Can you work these out from the model? Positions are in its coordinate system, mm. A direction names the side the tool comes from. Coordinates: 2 decimals unless noted, no trailing zeros. Order: outer loops, then holes, each group sorted by start corner. A loop starts at its lowest first (then second) coordinate and runs counter-clockwise, first axis right, second up. Notation, with made-up numbers: M 70,-11 L 80,-11 A13 cw 80,9 Z; hole C 40.25,76 d10. An arc over 180 degrees is marked long. Answer as CSV lines item,"result". Start each with the question number.
1. On a 3-axis mill with a long thin cutter (end or side, diameter ignored), from which of +Z, -Z, +X, -X, +Y, -Y can I reach the whole of each face in a straight line? I mean faces 5 (the face through (-0.631, -1.479, 92.056)), 6 (the face through (-55, -3, 40)), 7 (the face through (-121.908, -1.479, 1.504)). Say none if no direction works.
2. If we section it at D-D (z = 98): List the corners of the cut face in (x, y) for me, plus the area to 3 significant figures.
3. If we section it at A-A (z = 38): List the corners of the cut face in (x, y) for me, plus the area to 3 significant figures.
4. If we section it at C-C (x = -72): List the corners of the cut face in (y, z) for me.
5. Will these pins go through, and if not, where does the flat tip stop? pin 1 (1.5 mm diameter, centred on y = -2, z = 54.5, fed in from +X); pin 2 (1.5 mm diameter, centred on y = -1.5, z = 49, fed in from -X); pin 3 (1.5 mm diameter, centred on y = -2, z = 15.5, fed in from -X).
6. If we mould it in two halves opening along X, with no side actions, what happens to faces 1 (the face through (12.443, -1.479, 67.745)), 2 (the face through (-55, 0, 40)), 3 (the face through (-154.63, -1.48, 7.35)), 4 (the face through (45.943, -1.479, 87.404))? For each: released by +X, released by -X, zero draft, split by the parting line, or undercut.
7. I need wall thicknesses on line 1 along X through (y, z) = (-2, 72); line 2 along X through (y, z) = (-1.35, 34); line 3 along X through (y, z) = (-1, 64.5). Which ranges of each line are inside material? Lowest first, please. Write a range as from..to.
```python
from build123d import *

# Parameters (mm, degrees)
F1_DEPTH = 3


with BuildPart() as f1:
    # F0 (on Front) → F1 (new body)
    with BuildSketch(Plane.XZ):
        with BuildLine():
            Line((-20, 0), (-5, 0))
            ThreePointArc((-5, 0), (-1.464466, 1.464466), (0, 5))
            Line((0, 5), (0, 60))
            Line((0, 60), (25.2391, 75.709675))
            ThreePointArc((25.2391, 75.709675), (39.261161, 56.50437), (57.673644, 71.552373))
            Line((57.673644, 71.552373), (57.576732, 71.481567))
            Line((57.576732, 71.481567), (33.979088, 103.779418))
            Line((33.979088, 103.779418), (29.703019, 111.034036))
            Line((29.703019, 111.034036), (25.755882, 103.779418))
            Line((25.755882, 103.779418), (20.821964, 111.527428))
            Line((20.821964, 111.527428), (18.203917, 103.779418))
            Line((18.203917, 103.779418), (-20, 80))
            Line((-20, 80), (-120, 80))
            Line((-120, 80), (-132.250323, 93.696277))
            ThreePointArc((-132.250323, 93.696277), (-139.249154, 95.394938), (-143.333333, 89.462944))
            Line((-143.333333, 89.462944), (-143.333333, 9.462944))
            Line((-143.333333, 9.462944), (-156.787529, 25.438112))
            ThreePointArc((-156.787529, 25.438112), (-158.470845, 26.310515), (-160.278011, 25.737113))
            Line((-160.278011, 25.737113), (-164.137305, 22.486838))
            ThreePointArc((-164.137305, 22.486838), (-165.009708, 20.803522), (-164.436306, 18.996356))
            Line((-164.436306, 18.996356), (-144.540306, -4.627645))
            ThreePointArc((-144.540306, -4.627645), (-137.506096, -6.502206), (-133.333333, -0.53713))
            Line((-133.333333, -0.53713), (-133.333333, 82.907007))
            Line((-133.333333, 82.907007), (-123.333333, 71.726667))
            Line((-123.333333, 71.726667), (-123.333333, 5))
            ThreePointArc((-123.333333, 5), (-121.868867, 1.464466), (-118.333333, 0))
            Line((-118.333333, 0), (-103.333333, 0))
            Line((-103.333333, 0), (-103.333333, 25))
            Line((-103.333333, 25), (-100.333333, 25))
            Line((-100.333333, 25), (-100.333333, 0))
            Line((-100.333333, 0), (-23, 0))
            Line((-23, 0), (-23, 25))
            Line((-23, 25), (-20, 25))
            Line((-20, 25), (-20, 0))
        make_face()
    extrude(amount=F1_DEPTH)


solid = f1.part
```
Solved:
1,face 5,"+Z, +Y, -Y"
1,face 6,"+Z, -Z, +X, -X, -Y"
1,face 7,"-Z, +Y, -Y"
2,outline,"M 8.92,-3 L 38.2,-3 L 38.2,0 L 8.92,0 Z"
2,area,"87.8 mm²"
3,outline,"M -143.33,-3 L -133.33,-3 L -133.33,0 L -143.33,0 Z; M -123.33,-3 L 0,-3 L 0,0 L -123.33,0 Z"
3,area,"400 mm²"
4,outline,"M -3,0 L 0,0 L 0,80 L -3,80 Z"
5,pin 1,"x = 0"
5,pin 2,"x = -143.33"
5,pin 3,"x = -162.12"
6,face 1,"undercut"
6,face 2,"zero draft"
6,face 3,"released by -X"
6,face 4,"released by +X"
7,line 1,"-143.33..-133.33, -123.58..19.28, 24.99..57.2"
7,line 2,"-143.33..-133.33, -123.33..0"
7,line 3,"-143.33..-133.33, -123.33..7.23, 27.2..55.49"
